Work out the finished part from the listing and answer in its coordinate system (mm). Face numbers are marked on the shaded views. Give positions to 0.01 mm unless a question says otherwise; leave off trailing zeros. Write each loop counter-clockwise with the first axis right and the second up, starting at its lowest first coordinate (ties: lowest second). Pieces come first, ordered by that corner, then holes. Notation, with made-up numbers: (-12, 33.5) - (3, 33.5) arc R22 cw to (3, 46.5) - close; hole circle Ø10 at (-4, 8). An arc over 180 degrees is marked (long way). Write each question's results on one line, items separated by ' | '. Start each with the question number.
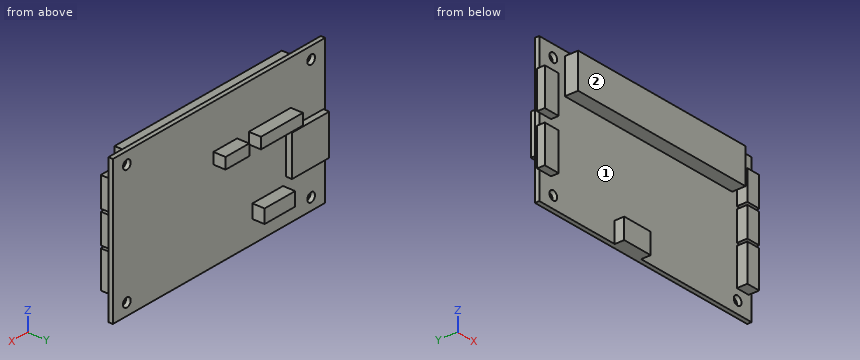
from build123d import *

# Parameters (mm, degrees)
SKETCH2_W           = 87
SKETCH2_H           = 50.18
SKETCH2_R           = 1.575
BOSS_EXTRUDE2_DEPTH = 1.55
SKETCH3_W           = 15.26
SKETCH3_H           = 14.07
BOSS_EXTRUDE3_DEPTH = 2.05
SKETCH4_W           = 17.2
SKETCH4_H           = 3.85
SKETCH4_W_2         = 9.7
SKETCH4_W_3         = 12.5
SKETCH4_H_2         = 4.75
BOSS_EXTRUDE4_DEPTH = 4.25
SKETCH7_W           = 68.55
SKETCH7_H           = 12.2
BOSS_EXTRUDE5_DEPTH = 4.65
SKETCH10_W          = 10.85
SKETCH10_H          = 7.15
BOSS_EXTRUDE6_DEPTH = 3.34
SKETCH11_W          = 5.7
SKETCH11_H          = 13
BOSS_EXTRUDE7_DEPTH = 2.7
SKETCH15_W          = 4.87
SKETCH15_H          = 10.25
SKETCH15_H_2        = 12.85
BOSS_EXTRUDE9_DEPTH = 3.68


with BuildPart() as part:
    # Sketch2 → Boss-Extrude2 (new body)
    with BuildSketch(Plane(origin=(0, 0, 0), x_dir=(1, 0, 0), z_dir=(0, 1, 0))):
        with Locations((-0.010528039, -0.006072379)):
            Rectangle(SKETCH2_W, SKETCH2_H)
        with Locations(Location((-37.760528039, 20.948927621, 0), (0, 0, 90))):
            Circle(SKETCH2_R, mode=Mode.SUBTRACT)
        with Locations(Location((-37.760528039, -20.948927621, 0), (0, 0, 90))):
            Circle(SKETCH2_R, mode=Mode.SUBTRACT)
        with Locations(Location((37.760528039, -20.948927621, 0), (0, 0, 90))):
            Circle(SKETCH2_R, mode=Mode.SUBTRACT)
        with Locations(Location((37.760528039, 20.948927621, 0), (0, 0, 90))):
            Circle(SKETCH2_R, mode=Mode.SUBTRACT)
    extrude(amount=BOSS_EXTRUDE2_DEPTH)

    # Sketch3 → Boss-Extrude3 (add)
    with BuildSketch(Plane(origin=(0, 1.55, 0), x_dir=(1, 0, 0), z_dir=(0, 1, 0))):
        with Locations((-35.130528039, 3.298927621)):
            Rectangle(SKETCH3_W, SKETCH3_H)
    extrude(amount=BOSS_EXTRUDE3_DEPTH)

    # Sketch4 → Boss-Extrude4 (add)
    with BuildSketch(Plane(origin=(0, 1.55, 0), x_dir=(1, 0, 0), z_dir=(0, 1, 0))):
        with Locations((-20.810528039, -7.871072379)):
            Rectangle(SKETCH4_W, SKETCH4_H)
        with Locations((-2.560528039, -7.871072379)):
            Rectangle(SKETCH4_W_2, SKETCH4_H)
        with Locations((-19.960528039, 15.008927621)):
            Rectangle(SKETCH4_W_3, SKETCH4_H_2)
    extrude(amount=BOSS_EXTRUDE4_DEPTH)

    # Sketch7 → Boss-Extrude5 (add)
    with BuildSketch(Plane(origin=(0, 0, 0), x_dir=(-1, 0, 0), z_dir=(0, -1, 0))):
        with Locations((-1.25778805, -17.316072379)):
            Rectangle(SKETCH7_W, SKETCH7_H)
    extrude(amount=BOSS_EXTRUDE5_DEPTH)

    # Sketch10 → Boss-Extrude6 (add)
    with BuildSketch(Plane.XZ):
        with Locations((-7.185528039, -21.508927621)):
            Rectangle(SKETCH10_W, SKETCH10_H)
    extrude(amount=BOSS_EXTRUDE6_DEPTH)

    # Sketch11 → Boss-Extrude7 (add)
    with BuildSketch(Plane.XZ):
        with Locations((-41.560528039, 8.346072379)):
            Rectangle(SKETCH11_W, SKETCH11_H)
        with Locations((-41.560528039, -9.053927621)):
            Rectangle(SKETCH11_W, SKETCH11_H)
    extrude(amount=BOSS_EXTRUDE7_DEPTH)

    # Sketch15 → Boss-Extrude9 (add)
    with BuildSketch(Plane.XZ):
        with Locations((39.867059602, 12.730529287)):
            Rectangle(SKETCH15_W, SKETCH15_H)
        with Locations((39.867059602, 1.580529287)):
            Rectangle(SKETCH15_W, SKETCH15_H)
        with Locations((39.867059602, -10.869470713)):
            Rectangle(SKETCH15_W, SKETCH15_H_2)
    extrude(amount=BOSS_EXTRUDE9_DEPTH)


solid = part.part
Q1. Given pin 1 (10 mm diameter, centred on x = 0.5, z = -10, fed in from -Y); pin 2 (1.3 mm diameter, centred on y = 3.5, z = -15, fed in from -X); pin 3 (3.5 mm diameter, centred on x = -21.5, y = 3.5, fed in from +Z); pin 4 (1.4 mm diameter, centred on x = -40.5, y = -0.5, fed in from -Z), each flat-ended and moving along its own axis, determine where each tip first touches the part or whether it passes through.
Q2. The mould has two halves that part along X. Classify the marked faces 1 and 2: pulls with the +X half, pulls with the -X half, needs draft (parallel to the pull), parting line crosses it, or undercut.
Q3. A cutting plane is placed at A-A, the plane y = -1.25. Write down the section's boundary in (x, z).
Q4. A cutting plane is placed at B-B, the plane z = -9.5. Write down the section's boundary in (x, y).
Q5. A cutting plane is placed at D-D, the plane z = 17. Write down the section's boundary in (x, y), and give its area (3 significant figures).
Q6. Consider L1, parallel to Z at x = -10, y = -0.5; L2, parallel to X at y = -1.75, z = -13.5; L3, parallel to X at y = -2.25, z = 15.5. Determine where each line is inside the solid, lowest interval first.
Q7. A cutting plane is placed at C-C, the plane x = 28. Write down the section's boundary in (y, z).
Result:
1) pin 1: stops at y = 0 | pin 2: stops at x = -26.21 | pin 3: stops at z = 9.8 | pin 4: stops at z = -25.08
2) face 1: undercut | face 2: needs draft
3) outline: (-44.41, -15.55) - (-38.71, -15.55) - (-38.71, -2.55) - (-44.41, -2.55) - close; (-44.41, 1.85) - (-38.71, 1.85) - (-38.71, 14.85) - (-44.41, 14.85) - close; (-33.02, 11.22) - (35.53, 11.22) - (35.53, 23.42) - (-33.02, 23.42) - close; (-12.61, -25.08) - (-1.76, -25.08) - (-1.76, -17.93) - (-12.61, -17.93) - close; (37.43, -17.29) - (42.3, -17.29) - (42.3, -4.44) - (37.43, -4.44) - close; (37.43, -3.54) - (42.3, -3.54) - (42.3, 6.71) - (37.43, 6.71) - close; (37.43, 7.61) - (42.3, 7.61) - (42.3, 17.86) - (37.43, 17.86) - close
4) outline: (-44.41, -2.7) - (-38.71, -2.7) - (-38.71, 0) - (37.43, 0) - (37.43, -3.68) - (42.3, -3.68) - (42.3, 0) - (43.49, 0) - (43.49, 1.55) - (-27.5, 1.55) - (-27.5, 3.6) - (-42.76, 3.6) - (-42.76, 1.55) - (-43.51, 1.55) - (-43.51, 0) - (-44.41, 0) - close
5) outline: (-43.51, 0) - (-33.02, 0) - (-33.02, -4.65) - (35.53, -4.65) - (35.53, 0) - (37.43, 0) - (37.43, -3.68) - (42.3, -3.68) - (42.3, 0) - (43.49, 0) - (43.49, 1.55) - (-43.51, 1.55) - close | area: 472 mm2
6) L1: z = -25.08 to -17.93, 11.22 to 23.42 | L2: x = -44.41 to -38.71, 37.43 to 42.3 | L3: x = -33.02 to 35.53, 37.43 to 42.3
7) outline: (-4.65, 11.22) - (0, 11.22) - (0, -25.08) - (1.55, -25.08) - (1.55, 25.1) - (0, 25.1) - (0, 23.42) - (-4.65, 23.42) - close
